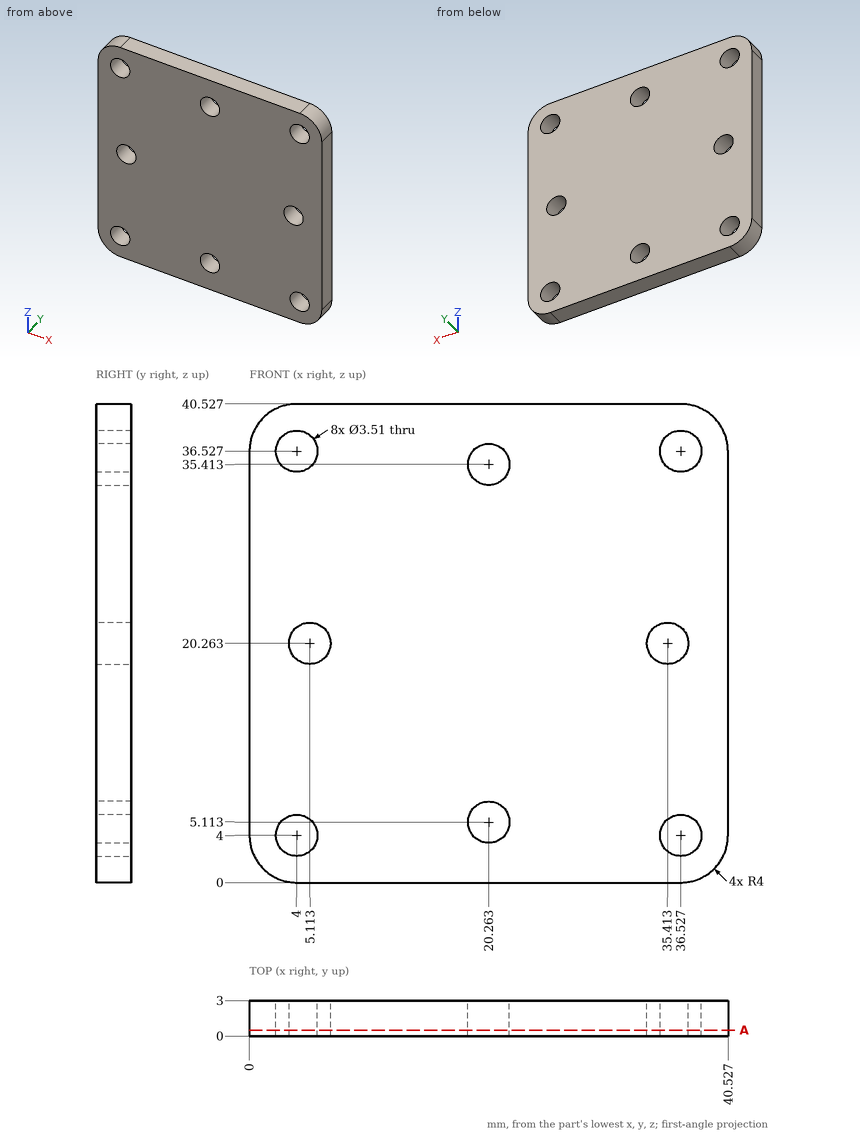
Here's the drawing with two shaded views (mm, measured from the low corner). I have some questions. Coordinates: 2 decimals unless noted, no trailing zeros.
Item 1: Will this pin go through, and if not, where does the flat tip stop? pin 1 (4.5 mm diameter, centred on x = 4, z = 36.53, fed in from -Y).
Item 2: If I drill on line 1 (X direction, y = 2.6, z = 36.5) (1 decimal); line 2 (Z direction, x = 2.5, y = 2.25) (1 decimal); line 3 (Z direction, x = 36, y = 0.7) (1 decimal), over which ranges is the centre line in solid material (lowest first)?
Item 3: I want a section at A-A on y = 0.5. Count the separate pieces of the cut face and the enclosed holes in it, and give its area (3 significant figures).
Findings below:
1. pin 1: stops at y = 0
2. line 1: x = 0 to 2.2, 5.8 to 18.9, 21.6 to 34.8, 38.3 to 40.5
2. line 2: z = 0.3 to 3.1, 4.9 to 35.6, 37.4 to 40.2
2. line 3: z = 0 to 2.3, 5.7 to 18.6, 21.9 to 34.9, 38.2 to 40.5
3. separate pieces: 1
3. enclosed holes: 8
3. area: 1,550 mm2
